Input: part model. Units: mm. Frame: model coordinates. Face numbers are marked on the shaded views. A direction names the side the tool comes from. Coordinates: 2 decimals unless noted, no trailing zeros. Write each loop counter-clockwise with the first axis right and the second up, starting at its lowest first coordinate (ties: lowest second). Pieces come first, ordered by that corner, then holes. Notation, with made-up numbers: (4, -10.5) - (28, -10.5) arc R19 ccw to (28, 11.5) - close; hole circle Ø8 at (85, -4.5). An arc over 180 degrees is marked (long way). One line per question, with ' | ' between items. Start each with the question number.
1) Section query B-B on y = 12.7. Give the number of separate pieces and of enclosed holes in the cut face, and give its area (3 significant figures).
2) Section query C-C on y = 20.32. Return loops of the section in (x, z), and give its area (3 significant figures).
3) Section query A-A on z = 45.72. Return loops of the section in (x, y).
4) Line query: line 1 (Y direction, x = 92.71, z = 93.3); line 2 (Y direction, x = -2.45, z = 15.24); line 3 (Y direction, x = 92, z = 98). Output: solid intervals per line, ascending.
5) Reachability of the marked faces 1, 2 and 3 from +Z, -Z, +X, -X, +Y, -Y: full face, straight path, thin tool, end or side. Return the list, or none.
6) Draft query along Y for the marked faces 4, 5, 6 and 7. Return one class per face: released by +Y, released by -Y, zero draft, split by the parting line, or undercut.
7) Section query D-D on z = 30.48. Return loops of the section in (x, y), and give its area (3 significant figures).
8) First-contact query: P1, Ø3, axis at x = 92.5, y = 21.5, coming from the +Z side; P2, Ø5.5, axis at x = 92.71, y = 5.08, coming from the -Z side; P3, Ø1.8, axis at y = 11.5, z = 46.5, coming from the -X side. Flat tips, straight axial feed; report the tip coordinate or a pass-through.
```python
from build123d import *

# Parameters (mm, degrees)
BOSS_EXTRUDE1_DEPTH     = 25.4
SKETCH4_R               = 3.302
CUT_EXTRUDE2_DEPTH      = 7.62
SKETCH2_R               = 1.5875
SKETCH2_R_2             = 3.302
CUT_EXTRUDE3_DEPTH      = 7.62
SKETCH6_W               = 121.92
SKETCH6_H               = 12.7
BOSS_EXTRUDE2_DEPTH     = 7.62
CUT_EXTRUDE4_DEPTH      = 3.81
SKETCH10_R              = 2.921
CUT_EXTRUDE5_DEPTH      = 3.048
SKETCH11_R              = 1.5875
CUT_EXTRUDE6_DEPTH      = 96.25
CUT_EXTRUDE7_REACH      = 101.06
SKETCH12_W              = 8.89
SKETCH12_H              = 20.32
CUT_EXTRUDE8_DEPTH      = 1
CUT_EXTRUDE8_DEPTH_BACK = 122.92
SKETCH15_R              = 1.651
CUT_EXTRUDE9_DEPTH      = 8.62
SKETCH16_R              = 2.921
CUT_EXTRUDE10_DEPTH     = 3.048
SKETCH17_W              = 46.323198875
SKETCH17_H              = 88.058880532
CUT_EXTRUDE11_DEPTH     = 51.8


with BuildPart() as part:
    # Sketch1 → Boss-Extrude1 (new body)
    with BuildSketch(Plane(origin=(0, 0, 0), x_dir=(1, 0, 0), z_dir=(0, 1, 0))):
        with BuildLine():
            Line((0, 0), (0, -59.69))
            ThreePointArc((0, -59.69), (9.299359697, -82.140640303), (31.75, -91.44))
            Line((31.75, -91.44), (69.85, -91.44))
            ThreePointArc((69.85, -91.44), (92.300640303, -82.140640303), (101.6, -59.69))
            Line((101.6, -59.69), (101.6, 0))
            Line((101.6, 0), (114.3, 0))
            Line((114.3, 0), (114.3, -99.06))
            Line((114.3, -99.06), (-7.62, -99.06))
            Line((-7.62, -99.06), (-7.62, 0))
            Line((-7.62, 0), (0, 0))
        make_face()
    extrude(amount=BOSS_EXTRUDE1_DEPTH)

    # Sketch4 → Cut-Extrude2 (cut)
    with BuildSketch(Plane.ZY.offset(-101.6)):
        with Locations((30.48, 12.7)):
            Circle(SKETCH4_R)
    extrude(amount=-CUT_EXTRUDE2_DEPTH, mode=Mode.SUBTRACT)

    # Sketch2 → Cut-Extrude3 (cut)
    with BuildSketch(Plane(origin=(0, 0, 0), x_dir=(0, 0, -1), z_dir=(1, 0, 0))):
        with Locations((-15.24, 12.7)):
            Circle(SKETCH2_R)
        with Locations((-45.72, 12.7)):
            Circle(SKETCH2_R)
        with Locations((-30.48, 12.7)):
            Circle(SKETCH2_R_2)
    extrude(amount=-CUT_EXTRUDE3_DEPTH, mode=Mode.SUBTRACT)

    # Sketch6 → Boss-Extrude2 (add)
    with BuildSketch(Plane.XY.offset(99.06)):
        with Locations((53.34, 31.75)):
            Rectangle(SKETCH6_W, SKETCH6_H)
        with Locations((53.34, -6.35)):
            Rectangle(SKETCH6_W, SKETCH6_H)
    extrude(amount=-BOSS_EXTRUDE2_DEPTH)

    # Sketch7 → Cut-Extrude4 (cut)
    with BuildSketch(Plane.XY.offset(99.06)):
        Polygon((12.284426472, 29.21), (9.901413236, 33.3375), (5.135386764, 33.3375), (2.752373528, 29.21), (5.135386764, 25.0825), (9.901413236, 25.0825), align=None)
        Polygon((103.724426472, -3.81), (101.341413236, 0.3175), (96.575386764, 0.3175), (94.192373528, -3.81), (96.575386764, -7.9375), (101.341413236, -7.9375), align=None)
    extrude(amount=-CUT_EXTRUDE4_DEPTH, mode=Mode.SUBTRACT)

    # Sketch10 → Cut-Extrude5 (cut)
    with BuildSketch(Plane.ZY.offset(7.62)):
        with Locations((15.24, 12.7)):
            Circle(SKETCH10_R)
        with Locations((45.72, 12.7)):
            Circle(SKETCH10_R)
    extrude(amount=-CUT_EXTRUDE5_DEPTH, mode=Mode.SUBTRACT)

    # Sketch11 → Cut-Extrude6 (cut, through all)
    with BuildSketch(Plane.XY.offset(95.25)):
        with Locations((7.5184, 29.21)):
            Circle(SKETCH11_R)
        with Locations((98.9584, -3.81)):
            Circle(SKETCH11_R)
    extrude(amount=-CUT_EXTRUDE6_DEPTH, mode=Mode.SUBTRACT)

    # Sketch12 → Cut-Extrude7 (cut, up to next)
    with BuildSketch(Plane.XY.offset(99.06), mode=Mode.PRIVATE) as cut_extrude7_sk1:
        with Locations((62.8396, 12.7)):
            Rectangle(SKETCH12_W, SKETCH12_H)
    cut_extrude7_tool1 = extrude(cut_extrude7_sk1.sketch, amount=-CUT_EXTRUDE7_REACH, mode=Mode.PRIVATE) & part.part
    add(cut_extrude7_tool1.solids().sort_by_distance((62.8396, 12.7, 99.06))[0], mode=Mode.SUBTRACT)

    # Sketch14 → Cut-Extrude8 (cut, two sides)
    with BuildSketch(Plane.ZY.offset(7.62)) as cut_extrude8_sk:
        with BuildLine():
            Line((14.426351463, 25.4), (0, 25.4))
            Line((0, 25.4), (0, 0))
            Line((0, 0), (14.426351463, 0))
            ThreePointArc((14.426351463, 0), (6.276222595, 12.7), (14.426351463, 25.4))
        make_face()
    extrude(amount=CUT_EXTRUDE8_DEPTH, mode=Mode.SUBTRACT)
    extrude(cut_extrude8_sk.sketch, amount=-CUT_EXTRUDE8_DEPTH_BACK, mode=Mode.SUBTRACT)

    # Sketch15 → Cut-Extrude9 (cut, through all)
    with BuildSketch(Plane(origin=(0, 0, 91.44), x_dir=(-1, 0, 0), z_dir=(0, 0, -1))):
        with Locations((-92.71, 20.32)):
            Circle(SKETCH15_R)
        with Locations((-92.71, 5.08)):
            Circle(SKETCH15_R)
    extrude(amount=-CUT_EXTRUDE9_DEPTH, mode=Mode.SUBTRACT)

    # Sketch16 → Cut-Extrude10 (cut)
    with BuildSketch(Plane.XY.offset(99.06)):
        with Locations((92.71, 20.32)):
            Circle(SKETCH16_R)
        with Locations((92.71, 5.08)):
            Circle(SKETCH16_R)
    extrude(amount=-CUT_EXTRUDE10_DEPTH, mode=Mode.SUBTRACT)

    # Sketch17 → Cut-Extrude11 (cut, through all)
    with BuildSketch(Plane(origin=(0, 38.1, 0), x_dir=(1, 0, 0), z_dir=(0, 1, 0))):
        with Locations((91.138400563, -47.410559734)):
            Rectangle(SKETCH17_W, SKETCH17_H)
    extrude(amount=-CUT_EXTRUDE11_DEPTH, mode=Mode.SUBTRACT)


solid = part.part
```
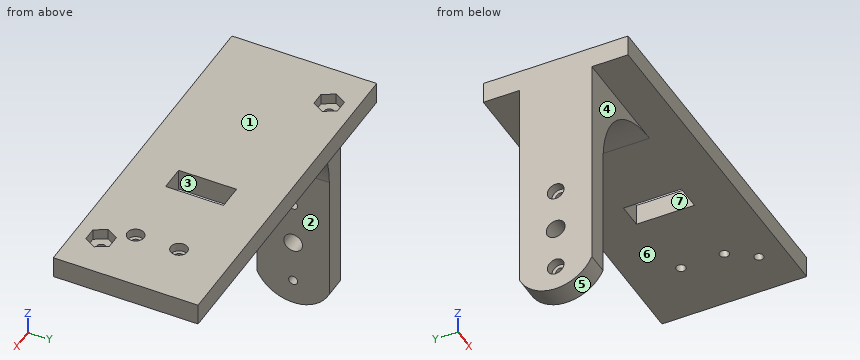
Answer key:
1) separate pieces: 5 | enclosed holes: 0 | area: 1,610 mm²
2) outline: (-7.62, 8.54) - (0, 8.54) - (0, 59.69) arc R31.75 cw to (31.75, 91.44) - (58.39, 91.44) - (58.39, 99.06) - (-7.62, 99.06) - close; (67.28, 91.44) - (91.06, 91.44) - (91.06, 96.01) - (89.79, 96.01) - (89.79, 99.06) - (67.28, 99.06) - close; (94.36, 91.44) - (114.3, 91.44) - (114.3, 99.06) - (95.63, 99.06) - (95.63, 96.01) - (94.36, 96.01) - close | area: 1,680 mm²
3) outline: (-7.62, 0) - (0, 0) - (0, 11.11) - (-4.57, 11.11) - (-4.57, 9.78) - (-7.62, 9.78) - close; (-7.62, 15.62) - (-4.57, 15.62) - (-4.57, 14.29) - (0, 14.29) - (0, 25.4) - (-7.62, 25.4) - close
4) line 1: -12.7 to 3.43, 6.73 to 18.67, 21.97 to 38.1 | line 2: 0 to 11.11, 14.29 to 25.4 | line 3: -12.7 to 2.25, 7.91 to 17.49, 23.15 to 38.1
5) face 1: +Z, +X, -X, +Y, -Y | face 2: -Z, +X, +Y, -Y | face 3: +Z, -Z
6) face 4: released by -Y | face 5: split by the parting line | face 6: zero draft | face 7: undercut
7) outline: (-7.62, 0) - (0, 0) - (0, 9.4) - (-7.62, 9.4) - close; (-7.62, 16) - (0, 16) - (0, 25.4) - (-7.62, 25.4) - close | area: 143 mm²
8) P1: z = 96.01 | P2: z = 91.44 | P3: x = -4.57
